Answer from the drawing. Dimensions are ordinates in mm from the lowest x, y and z of the part. A direction names the side the tool comes from. Give positions to 0.01 mm unless a question says otherwise; leave off trailing zeros. Write each loop counter-clockwise with the first axis right and the second up, starting at its lowest first coordinate (ties: lowest second). Pieces come first, ordered by that corner, then holes. Notation, with made-up numbers: (73.5, -13) - (103.5, -13) arc R20 cw to (103.5, 4) - close; hole circle Ø10 at (-9, 79.5). An arc over 180 degrees is marked (long way). Answer as a JSON object with one key per item and string values. Group by question number.
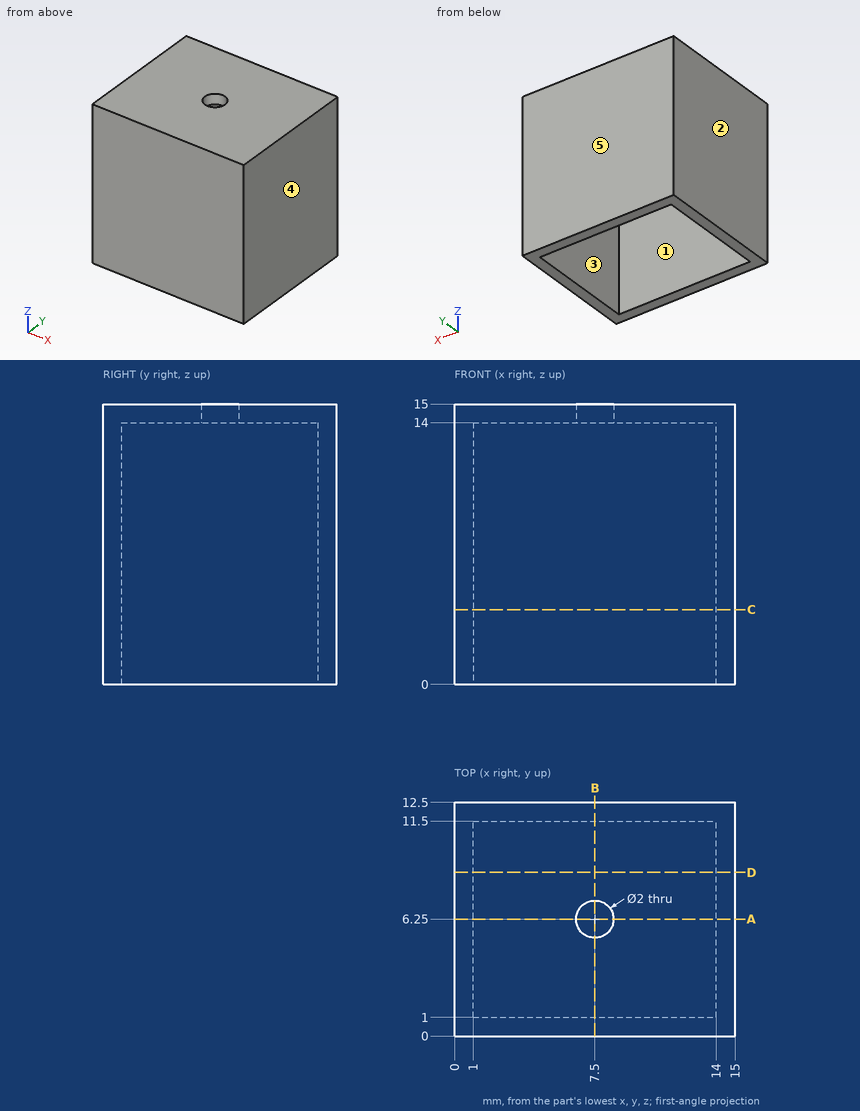
1) Find section C-C, the plane z = 4. Write down the section's boundary in (x, y).
2) A flat-ended cylindrical pin translates along its axis: pin 1 Ø3 at (x, y) = (7.5, 6.25) entering from -Z. Find the tip coordinate at first contact, or state that the pin passes through.
3) Which of the six approach directions +Z, -Z, +X, -X, +Y, -Y give full straight-line access (tool end or side, diameter ignored) to the marked faces 1 and 2?
4) Find the intervals of material crossed by line 1 (Y direction, x = 2.75, z = 13.5); line 2 (X direction, y = 4.75, z = 0.5); line 3 (Y direction, x = 7.5, z = 14.8), in increasing order. Write a range as [from, to].
5) Find section A-A, the plane y = 6.25. Write down the section's boundary in (x, z), and give its area (3 significant figures).
6) Find section D-D, the plane y = 8.75. Write down the section's boundary in (x, z), and give its area (3 significant figures).
7) For a pull along Y with two mould halves and no side action, classify the marked faces 3, 4 and 5 as released by +Y, released by -Y, zero draft, split by the parting line, or undercut.
8) Find section B-B, the plane x = 7.5. Write down the section's boundary in (y, z).
Values follow:
{
 "1": {"outline": "(0, 0) - (15, 0) - (15, 12.5) - (0, 12.5) - close; hole (1, 1) - (14, 1) - (14, 11.5) - (1, 11.5) - close"},
 "2": {"pin 1": "stops at z = 14"},
 "3": {"face 1": "-Z", "face 2": "+Z, -Z, -X, +Y, -Y"},
 "4": {"line 1": "y = [0, 1], [11.5, 12.5]", "line 2": "x = [0, 1], [14, 15]", "line 3": "y = [0, 5.25], [7.25, 12.5]"},
 "5": {"outline": "(0, 0) - (1, 0) - (1, 14) - (6.5, 14) - (6.5, 15) - (0, 15) - close; (8.5, 14) - (14, 14) - (14, 0) - (15, 0) - (15, 15) - (8.5, 15) - close", "area": "41.0 mm2"},
 "6": {"outline": "(0, 0) - (1, 0) - (1, 14) - (14, 14) - (14, 0) - (15, 0) - (15, 15) - (0, 15) - close", "area": "43.0 mm2"},
 "7": {"face 3": "undercut", "face 4": "zero draft", "face 5": "released by +Y"},
 "8": {"outline": "(0, 0) - (1, 0) - (1, 14) - (5.25, 14) - (5.25, 15) - (0, 15) - close; (7.25, 14) - (11.5, 14) - (11.5, 0) - (12.5, 0) - (12.5, 15) - (7.25, 15) - close"}
}
